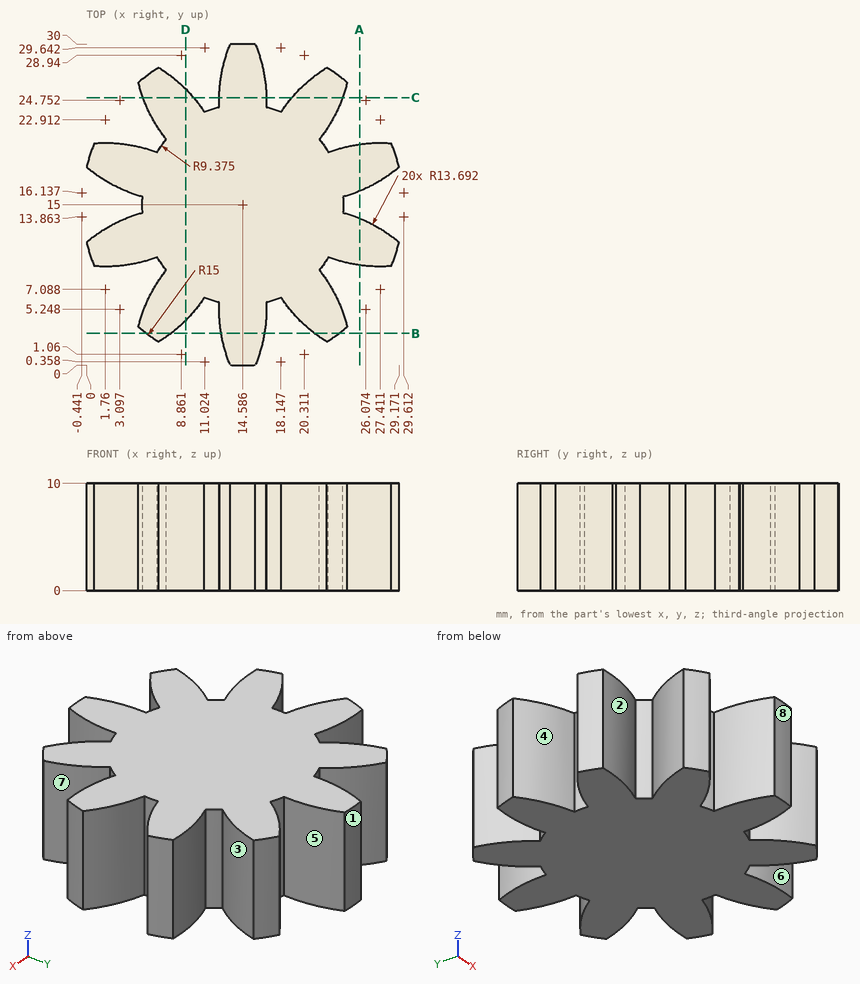
Part print with two shaded views. Sizes in mm from the minimum x, y, z corner. A direction names the side the tool comes from. Round coordinates to 2 decimals unless told otherwise and drop trailing zeros. Loops run counter-clockwise (first coordinate to the right, second up) from the corner with the lowest first, then second, coordinate; pieces in that order, holes last.
1. 3-axis set-ups, long thin cutter, end or side, ignore diameter. For the marked faces 1, 2, 3 and 4: which of +Z, -Z, +X, -X, +Y, -Y reach the whole face in a straight line?
Solutions:
face 1: +Z, -Z, +Y
face 2: +Z, -Z
face 3: +Z, -Z, +X
face 4: +Z, -Z, -X
2. Slice it at A-A (x = 25.5). Give the cut face in (y, z) (1 decimal).
Solutions:
outline: (9.4, 0) - (13.7, 0) - (13.7, 10) - (9.4, 10) - close; (16.3, 0) - (20.6, 0) - (20.6, 10) - (16.3, 10) - close
3. Two-plate mould, pull along X, no slides. Class the marked faces 5, 6, 7 and 8: pulls with the +X half, pulls with the -X half, needs draft (parallel to the pull), parting line crosses it, or undercut.
Solutions:
face 5: undercut
face 6: undercut
face 7: pulls with the +X half
face 8: parting line crosses it
4. Slice it at B-B (y = 3). Give the cut face in (x, z) (1 decimal).
Solutions:
outline: (5.6, 0) - (7.9, 0) - (7.9, 10) - (5.6, 10) - close; (12.6, 0) - (16.6, 0) - (16.6, 10) - (12.6, 10) - close; (21.3, 0) - (23.6, 0) - (23.6, 10) - (21.3, 10) - close
5. Slice it at D-D (x = 9.25). Give the cut face in (y, z), and give its area (3 significant figures).
Solutions:
outline: (4.19, 0) - (25.81, 0) - (25.81, 10) - (4.19, 10) - close
area: 216 mm2
6. Drill centre lines: line 1 along X through (y, z) = (27.5, 3) (1 decimal); line 2 along X through (y, z) = (5.5, 2.25) (1 decimal); line 3 along Y through (x, z) = (7.25, 9.75) (1 decimal). Where is each one in solid material? Low to high.
Solutions:
line 1: x = 6.3 to 7.2, 12.7 to 16.5, 22 to 22.9
line 2: x = 5.5 to 10.4, 12.4 to 16.8, 18.8 to 23.7
line 3: y = 2.5 to 8.6, 9.2 to 20.8, 21.4 to 27.5
7. Slice it at C-C (y = 25). Give the cut face in (x, z) (1 decimal).
Solutions:
outline: (5.3, 0) - (10, 0) - (10, 10) - (5.3, 10) - close; (12.4, 0) - (16.8, 0) - (16.8, 10) - (12.4, 10) - close; (19.2, 0) - (23.9, 0) - (23.9, 10) - (19.2, 10) - close
